Part model, mm, in its own coordinate system. Face numbers are marked on the shaded views. A direction names the side the tool comes from. Round coordinates to 2 decimals unless told otherwise and drop trailing zeros. Write each loop counter-clockwise with the first axis right and the second up, starting at its lowest first coordinate (ties: lowest second). Pieces come first, ordered by that corner, then holes. Notation, with made-up numbers: M -7,11.25 L 9,11.25 A25 cw 9,28.25 Z; hole C 26,-26.5 d8. An arc over 180 degrees is marked long. Use one line per item in the form item = value. Start each with the question number.
Item 1: Cut at D-D, the plane y = -17. Give the cut face in (x, z), then the cut area to 3 significant figures.
Item 2: Cut at C-C, the plane x = 0. Give the cut face in (y, z) (1 decimal), then the cut area to 3 significant figures.
Item 3: Probe L1, parallel to Y at x = 0, z = 0.6 (1 decimal); L2, parallel to Y at x = -0.25, z = 2; L3, parallel to Y at x = 7, z = 5.5. List the from-to ranges inside material, lowest first.
Item 4: Cut at A-A, the plane z = 2.75. Give the cut face in (x, y), then the cut area to 3 significant figures.
Item 5: Mould opens along Y. For the marked faces 3, 4 and 5 say: +Y half, -Y half, draft (parallel to the pull), parting line (faces both ways), or undercut.
Item 6: Flat gauge pin, fed straight in: pin 1 Ø8.5 at (x, y) = (-1, 2) entering from +Z. Where does the tip first touch, or does it go through?
Item 7: Which spindle directions (+Z, -Z, +X, -X, +Y, -Y) get a long thin tool onto all of the face, cutting with end or side? Do the marked faces 1 and 2. Say none if no direction does.
Item 8: Cut at B-B, the plane y = 0. Give the cut face in (x, z) (3 decimals), then the cut area to 3 significant figures.
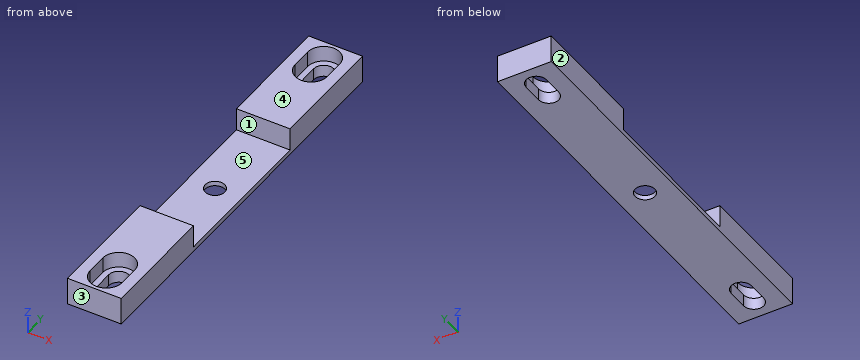
from build123d import *

# Parameters (mm, degrees)
SKETCH1_W                       = 17.272
SKETCH1_H                       = 127
BOSS_EXTRUDE1_DEPTH             = 8.89
F_1_4_0_25_DIAMETER_HOLE1_D     = 6.35
F_1_4_0_25_DIAMETER_HOLE1_DEPTH = 8.89
SKETCH5_W                       = 17.272
SKETCH5_H                       = 50.8
CUT_EXTRUDE1_DEPTH              = 7.366
CUT_EXTRUDE2_DEPTH              = 9.89
CUT_EXTRUDE3_DEPTH              = 5.08


with BuildPart() as part:
    # Sketch1 → Boss-Extrude1 (new body)
    with BuildSketch(Plane.XY):
        Rectangle(SKETCH1_W, SKETCH1_H)
    extrude(amount=BOSS_EXTRUDE1_DEPTH)

    # 1/4 (0.25) Diameter Hole1
    with Locations(Plane.XY.offset(8.89)):
        with Locations((0, 0)):
            Hole(F_1_4_0_25_DIAMETER_HOLE1_D / 2, depth=F_1_4_0_25_DIAMETER_HOLE1_DEPTH)

    # Sketch5 → Cut-Extrude1 (cut)
    with BuildSketch(Plane.XY.offset(8.89)):
        Rectangle(SKETCH5_W, SKETCH5_H)
    extrude(amount=-CUT_EXTRUDE1_DEPTH, mode=Mode.SUBTRACT)

    # Sketch13 → Cut-Extrude2 (cut, through all)
    with BuildSketch(Plane.XY.offset(8.89)):
        with BuildLine():
            Line((3.2385, 57.277), (3.2385, 50.673))
            ThreePointArc((3.2385, 50.673), (0, 47.4345), (-3.2385, 50.673))
            Line((-3.2385, 50.673), (-3.2385, 57.277))
            ThreePointArc((-3.2385, 57.277), (0, 60.5155), (3.2385, 57.277))
        make_face()
        with BuildLine():
            Line((3.2385, -57.277), (3.2385, -50.673))
            ThreePointArc((3.2385, -50.673), (0, -47.4345), (-3.2385, -50.673))
            Line((-3.2385, -50.673), (-3.2385, -57.277))
            ThreePointArc((-3.2385, -57.277), (0, -60.5155), (3.2385, -57.277))
        make_face()
    extrude(amount=-CUT_EXTRUDE2_DEPTH, mode=Mode.SUBTRACT)

    # Sketch14 → Cut-Extrude3 (cut)
    with BuildSketch(Plane.XY.offset(8.89)):
        with BuildLine():
            Line((-5.159375, 50.673), (-5.159375, 57.277))
            ThreePointArc((-5.159375, 57.277), (0, 62.436375), (5.159375, 57.277))
            Line((5.159375, 57.277), (5.159375, 50.673))
            ThreePointArc((5.159375, 50.673), (0, 45.513625), (-5.159375, 50.673))
        make_face()
        with BuildLine():
            Line((5.159375, -50.673), (5.159375, -57.277))
            ThreePointArc((5.159375, -57.277), (0, -62.436375), (-5.159375, -57.277))
            Line((-5.159375, -57.277), (-5.159375, -50.673))
            ThreePointArc((-5.159375, -50.673), (0, -45.513625), (5.159375, -50.673))
        make_face()
    extrude(amount=-CUT_EXTRUDE3_DEPTH, mode=Mode.SUBTRACT)


solid = part.part
Model answer:
q1.outline = M -8.64,0 L 8.64,0 L 8.64,1.52 L -8.64,1.52 Z
q1.area = 26.3 mm²
q2.outline = M -63.5,0 L -60.5,0 L -60.5,3.8 L -62.4,3.8 L -62.4,8.9 L -63.5,8.9 Z; M -47.4,0 L -3.2,0 L -3.2,1.5 L -25.4,1.5 L -25.4,8.9 L -45.5,8.9 L -45.5,3.8 L -47.4,3.8 Z; M 3.2,0 L 47.4,0 L 47.4,3.8 L 45.5,3.8 L 45.5,8.9 L 25.4,8.9 L 25.4,1.5 L 3.2,1.5 Z; M 60.5,0 L 63.5,0 L 63.5,8.9 L 62.4,8.9 L 62.4,3.8 L 60.5,3.8 Z
q2.area = 474 mm²
q3.L1 = -63.5 to -60.5, -47.4 to -3.2, 3.2 to 47.4, 60.5 to 63.5
q3.L2 = -63.5 to -60.51, -47.44 to -25.4, 25.4 to 47.44, 60.51 to 63.5
q3.L3 = -63.5 to -25.4, 25.4 to 63.5
q4.outline = M -8.64,-63.5 L 8.64,-63.5 L 8.64,-25.4 L -8.64,-25.4 Z; M -8.64,25.4 L 8.64,25.4 L 8.64,63.5 L -8.64,63.5 Z; hole M -3.24,-57.28 A3.24 ccw 3.24,-57.28 L 3.24,-50.67 A3.24 ccw -3.24,-50.67 Z; hole M -3.24,50.67 A3.24 ccw 3.24,50.67 L 3.24,57.28 A3.24 ccw -3.24,57.28 Z
q4.area = 1,160 mm²
q5.face_3 = -Y half
q5.face_4 = draft
q5.face_5 = undercut
q6.pin_1 = 1.52
q7.face_1 = +Z, +X, -X
q7.face_2 = +Z, -Z, -X, +Y, -Y
q8.outline = M -8.636,0 L -3.175,0 L -3.175,1.524 L -8.636,1.524 Z; M 3.175,0 L 8.636,0 L 8.636,1.524 L 3.175,1.524 Z
q8.area = 16.6 mm²
